Can you work these out from the model? Positions are in its coordinate system, mm. A direction names the side the tool comes from. Round coordinates to 2 decimals unless told otherwise and drop trailing zeros. Loops run counter-clockwise (first coordinate to the right, second up) from the corner with the lowest first, then second, coordinate; pieces in that order, holes last.
```python
from build123d import *

# Parameters (mm, degrees)
ESQUISSE1_W             = 48
ESQUISSE1_H             = 38
BOSS_EXTRU_1_DEPTH      = 7.5
ESQUISSE2_R             = 1.75
ENL_V_MAT_EXTRU_1_DEPTH = 7.5
ESQUISSE4_W             = 14
ESQUISSE4_H             = 15
ENL_V_MAT_EXTRU_2_DEPTH = 7.5


with BuildPart() as part:
    # Esquisse1 → Boss.-Extru.1 (new body)
    with BuildSketch(Plane.XY):
        Rectangle(ESQUISSE1_W, ESQUISSE1_H)
    extrude(amount=BOSS_EXTRU_1_DEPTH)

    # Esquisse2 → Enlèv. mat.-Extru.1 (cut)
    with BuildSketch(Plane.XY.offset(7.5)):
        with Locations((20.75, 15.25)):
            Circle(ESQUISSE2_R)
        with Locations((-20.75, 15.25)):
            Circle(ESQUISSE2_R)
        with Locations((20.75, -15.25)):
            Circle(ESQUISSE2_R)
        with Locations((-20.75, -15.25)):
            Circle(ESQUISSE2_R)
    extrude(amount=-ENL_V_MAT_EXTRU_1_DEPTH, mode=Mode.SUBTRACT)

    # Esquisse4 → Enlèv. mat.-Extru.2 (cut)
    with BuildSketch(Plane.XY.offset(7.5)):
        with Locations((17, 0)):
            Rectangle(ESQUISSE4_W, ESQUISSE4_H)
    extrude(amount=-ENL_V_MAT_EXTRU_2_DEPTH, mode=Mode.SUBTRACT)


solid = part.part
```
(1) We'd pull the mould along Y, two halves only. Please class faces 1 (the flat face through (0, 0, 0)), 2 (the flat face through (0, -19, 4)), 3 (the cylindrical face through (-22.04, -14.07, 3.8)): released by +Y, released by -Y, zero draft, split by the parting line, or undercut.
(2) Suppose I cut it at A-A (x = 18.5). Write out the boundary of the cut face in (y, z), then the cut area to 4 significant figures.
(3) For pin 1 (3 mm diameter, centred on x = 20.75, y = -15.25, fed in from -Z); pin 2 (1.5 mm diameter, centred on y = -5, z = 6, fed in from +X), each with a flat end and sliding along its axis, tell me the tip position at first contact or that it passes through.
(4) Suppose I cut it at D-D (x = -20.75). Write out the boundary of the cut face in (y, z), then the cut area to 4 significant figures.
(5) Which directions (+Z, -Z, +X, -X, +Y, -Y) give clear straight access to the entire face, cutting with the end or side of a thin tool? Please do faces 4 (the flat face through (-24, 0, 4)), 5 (the flat face through (17, 7.5, 4)).
(6) If I drill on line 1 (Y direction, x = -20.75, z = 2.75); line 2 (Y direction, x = 20.75, z = 3.75); line 3 (Y direction, x = 18, z = 3.5), over which ranges is the centre line in solid material (lowest first)?
(7) Suppose I cut it at B-B (y = 15.25). Write out the boundary of the cut face in (x, z).
(8) Suppose I cut it at C-C (z = 4). Write out the boundary of the cut face in (x, y).
Check result:
1. face 1: zero draft
1. face 2: released by -Y
1. face 3: undercut
2. outline: (-19, 0) - (-7.5, 0) - (-7.5, 7.5) - (-19, 7.5) - close; (7.5, 0) - (19, 0) - (19, 7.5) - (7.5, 7.5) - close
2. area: 172.5 mm2
3. pin 1: passes through
3. pin 2: stops at x = 10
4. outline: (-19, 0) - (-17, 0) - (-17, 7.5) - (-19, 7.5) - close; (-13.5, 0) - (13.5, 0) - (13.5, 7.5) - (-13.5, 7.5) - close; (17, 0) - (19, 0) - (19, 7.5) - (17, 7.5) - close
4. area: 232.5 mm2
5. face 4: +Z, -Z, -X, +Y, -Y
5. face 5: +Z, -Z, +X
6. line 1: y = -19 to -17, -13.5 to 13.5, 17 to 19
6. line 2: y = -19 to -17, -13.5 to -7.5, 7.5 to 13.5, 17 to 19
6. line 3: y = -19 to -7.5, 7.5 to 19
7. outline: (-24, 0) - (-22.5, 0) - (-22.5, 7.5) - (-24, 7.5) - close; (-19, 0) - (19, 0) - (19, 7.5) - (-19, 7.5) - close; (22.5, 0) - (24, 0) - (24, 7.5) - (22.5, 7.5) - close
8. outline: (-24, -19) - (24, -19) - (24, -7.5) - (10, -7.5) - (10, 7.5) - (24, 7.5) - (24, 19) - (-24, 19) - close; hole circle Ø3.5 at (-20.75, -15.25); hole circle Ø3.5 at (-20.75, 15.25); hole circle Ø3.5 at (20.75, -15.25); hole circle Ø3.5 at (20.75, 15.25)
